Input: part model. Units: mm. Frame: model coordinates. A direction names the side the tool comes from. Coordinates: 2 decimals unless noted, no trailing zeros. Write each loop counter-clockwise with the first axis right and the second up, starting at its lowest first coordinate (ties: lowest second). Pieces come first, ordered by that corner, then holes. Notation, with made-up numbers: (-39.75, -34.75) -> (8.25, -34.75) arc R29 cw to (8.25, 0.25) -> close; hole circle Ø5 at (2.25, 70.5). An arc over 180 degrees is marked (long way). One line per question, with ' | ' between items. Start each with the question number.
```python
from build123d import *

# Parameters (mm, degrees)
EXTRUDE_1_DEPTH     = 3.47
FILLET_1_R          = 2
MM_1_D              = 3
MM_1_CSINK_D        = 3.05
MM_1_CSINK_ANGLE    = 90
SKETCH_5_R          = 2.15
CUT_EXTRUDE_1_DEPTH = 2


with BuildPart() as part:
    # 草图1 → 凸台-拉伸1 (new body)
    with BuildSketch(Plane.XY):
        with BuildLine():
            Line((-25.5, -8), (-20, -8))
            Line((-20, -8), (-20, -10.5))
            ThreePointArc((-20, -10.5), (-17.5, -13), (-15, -10.5))
            Line((-15, -10.5), (-15, -8))
            Line((-15, -8), (15, -8))
            Line((15, -8), (15, -10.5))
            ThreePointArc((15, -10.5), (17.5, -13), (20, -10.5))
            Line((20, -10.5), (20, -8))
            Line((20, -8), (25.5, -8))
            Line((25.5, -8), (25.5, 8))
            Line((25.5, 8), (20, 8))
            Line((20, 8), (20, 10.5))
            ThreePointArc((20, 10.5), (17.5, 13), (15, 10.5))
            Line((15, 10.5), (15, 8))
            Line((15, 8), (-15, 8))
            Line((-15, 8), (-15, 10.5))
            ThreePointArc((-15, 10.5), (-17.5, 13), (-20, 10.5))
            Line((-20, 10.5), (-20, 8))
            Line((-20, 8), (-25.5, 8))
            Line((-25.5, 8), (-25.5, -8))
        make_face()
    extrude(amount=EXTRUDE_1_DEPTH)

    # 圆角1
    fillet_1_edges = [part.edges().sort_by_distance(p)[0] for p in [
        (25.5, 8, 1.735),
        (25.5, -8, 1.735),
        (20, -8, 1.735),
        (15, -8, 1.735),
        (-15, -8, 1.735),
        (-20, -8, 1.735),
        (-25.5, -8, 1.735),
        (-25.5, 8, 1.735),
        (-20, 8, 1.735),
        (-15, 8, 1.735),
        (15, 8, 1.735),
        (20, 8, 1.735),
    ]]
    fillet(fillet_1_edges, radius=FILLET_1_R)

    # 大小mm 暗销孔1 (through all)
    with Locations(Plane.XY.offset(3.47)):
        with Locations((-17.5, 10.5), (-17.5, -10.5), (17.5, -10.5), (17.5, 10.5)):
            CounterSinkHole(MM_1_D / 2, MM_1_CSINK_D / 2, counter_sink_angle=MM_1_CSINK_ANGLE)

    # 草图5 → 切除-拉伸1 (cut)
    with BuildSketch(Plane.XY.offset(3.47)):
        with Locations((-17.5, 10.5)):
            Circle(SKETCH_5_R)
        with Locations((17.5, 10.5)):
            Circle(SKETCH_5_R)
        with Locations((-17.5, -10.5)):
            Circle(SKETCH_5_R)
        with Locations((17.5, -10.5)):
            Circle(SKETCH_5_R)
    extrude(amount=-CUT_EXTRUDE_1_DEPTH, mode=Mode.SUBTRACT)


solid = part.part
```
1) Access query for faces 5 (the face through (18.4, 9.1, 1.47)), 6 (the face through (0, 8, 2)), 7 (the face through (23, 8, 2)). Directions: +Z, -Z, +X, -X, +Y, -Y. A direction counts if a zero-diameter tool reaches every point of the face in a straight line with its end or side. Return the directions, or none.
2) Pull-direction query (Y, two-part tool) for faces 1 (the face through (0, 0, 0)), 2 (the face through (0, -8, 2)), 3 (the face through (-16.51, 8.59, 2.48)), 4 (the face through (18.49, 8.59, 2.48)); classes: released by +Y, released by -Y, zero draft, split by the parting line, or undercut.
3) Ray query, line 1 (Y direction, x = 17.5, z = 2.5); line 2 (X direction, y = 11.5, z = 0.9); line 3 (Y direction, x = -9.5, z = 0.85). Return the intervals inside material, ascending.
4) Section A-A, the plane x = -17.5. Return loops of the section in (y, z), then the cut area to 3 significant figures.
5) Section B-B, the plane z = 2. Give the number of separate pieces and of enclosed holes in the cut face, then the cut area to 3 significant figures.
6) First-contact query: P1, Ø1, axis at x = -18.5, z = 2.5, coming from the +Y side; P2, Ø1.7, axis at x = -2.5, z = 2.5, coming from the +Y side. Flat tips, straight axial feed; report the tip coordinate or a pass-through.
Answer block:
1) face 5: +Z | face 6: +Z, -Z, +Y | face 7: +Z, -Z, +X, +Y
2) face 1: zero draft | face 2: released by -Y | face 3: undercut | face 4: undercut
3) line 1: y = -13 to -12.65, -8.35 to 8.35, 12.65 to 13 | line 2: x = -19.79 to -18.62, -16.38 to -15.21, 15.21 to 16.38, 18.62 to 19.79 | line 3: y = -8 to 8
4) outline: (-13, 0) -> (-12, 0) -> (-12, 1.47) -> (-12.65, 1.47) -> (-12.65, 3.47) -> (-13, 3.47) -> close; (-9, 0) -> (9, 0) -> (9, 1.47) -> (8.35, 1.47) -> (8.35, 3.47) -> (-8.35, 3.47) -> (-8.35, 1.47) -> (-9, 1.47) -> close; (12, 0) -> (13, 0) -> (13, 3.47) -> (12.65, 3.47) -> (12.65, 1.47) -> (12, 1.47) -> close | area: 64.2 mm2
5) separate pieces: 1 | enclosed holes: 4 | area: 851 mm2
6) P1: stops at y = 12.95 | P2: stops at y = 8
